Here's how the part is built. I have some questions about the finished solid (model axes, mm). Give positions to 0.01 mm unless a question says otherwise; leave off trailing zeros. Write each loop counter-clockwise with the first axis right and the second up, starting at its lowest first coordinate (ties: lowest second). Pieces come first, ordered by that corner, then holes. Notation, with made-up numbers: (48.25, -10) - (55.25, -10) arc R19 cw to (55.25, 8) - close; hole circle Ø5 at (-4, 16.5). An arc over 180 degrees is marked (long way). One line per item, written item: value. Start each with the question number.
1) I'm going to push flat-ended pins straight in: P1, Ø3, axis at y = 82.5, z = 0.5, coming from the +X side; P2, Ø2.5, axis at y = 65.5, z = 1.5, coming from the +X side; P3, Ø1.5, axis at x = 11, z = 3, coming from the +Y side. Where does each tip first touch, or does it pass through?
2) Imagine slicing it at A-A on z = 2.65. Write out the boundary of the cut face in (x, y).
3) Imagine slicing it at B-B on y = 16.5. Write out the boundary of the cut face in (x, z).
4) Imagine slicing it at C-C on x = -57. Write out the boundary of the cut face in (y, z), plus the area to 3 significant figures.
5) Please list where these lines run through material, in increasing order: L1, parallel to X at y = 4.5, z = 2.5; L2, parallel to X at y = 26.5, z = 2.9; L3, parallel to X at y = 55, z = 1.4. Write a range as [from, to].
6) Imagine slicing it at D-D on x = 2. Write out the boundary of the cut face in (y, z), plus the area to 3 significant figures.
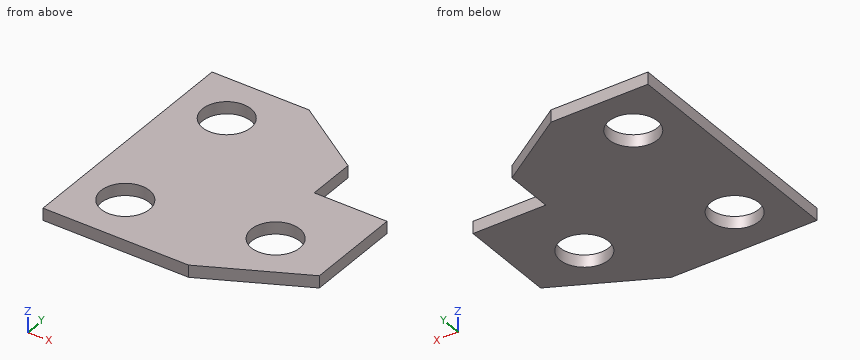
from build123d import *

# Parameters (mm, degrees)
SKETCH1_R           = 10
BOSS_EXTRUDE1_DEPTH = 5


with BuildPart() as part:
    # Sketch1 → Boss-Extrude1 (new body)
    with BuildSketch(Plane.XY):
        Polygon((-73.294117647, 93.764705882), (-73.294117647, -6.235294118), (-13.294117647, -6.235294118), (26.705882353, 13.764705882), (26.705882353, 53.764705882), (-3.294117647, 53.764705882), (-3.294117647, 73.764705882), (-33.294117647, 93.764705882), align=None)
        with Locations((-53.294117647, 73.764705882)):
            Circle(SKETCH1_R, mode=Mode.SUBTRACT)
        with Locations((-53.294117647, 13.764705882)):
            Circle(SKETCH1_R, mode=Mode.SUBTRACT)
        with Locations((1.705882353, 23.764705882)):
            Circle(SKETCH1_R, mode=Mode.SUBTRACT)
    extrude(amount=BOSS_EXTRUDE1_DEPTH)


solid = part.part
Numbers:
1. P1: x = -14.15
1. P2: x = -3.29
1. P3: y = 53.76
2. outline: (-73.29, -6.24) - (-13.29, -6.24) - (26.71, 13.76) - (26.71, 53.76) - (-3.29, 53.76) - (-3.29, 73.76) - (-33.29, 93.76) - (-73.29, 93.76) - close; hole circle Ø20 at (-53.29, 13.76); hole circle Ø20 at (-53.29, 73.76); hole circle Ø20 at (1.71, 23.76)
3. outline: (-73.29, 0) - (-62.91, 0) - (-62.91, 5) - (-73.29, 5) - close; (-43.68, 0) - (-5.17, 0) - (-5.17, 5) - (-43.68, 5) - close; (8.58, 0) - (26.71, 0) - (26.71, 5) - (8.58, 5) - close
4. outline: (-6.24, 0) - (4.48, 0) - (4.48, 5) - (-6.24, 5) - close; (23.05, 0) - (64.48, 0) - (64.48, 5) - (23.05, 5) - close; (83.05, 0) - (93.76, 0) - (93.76, 5) - (83.05, 5) - close
4. area: 314 mm^2
5. L1: [-73.29, -57.06], [-49.53, 8.18]
5. L2: [-73.29, -7.91], [11.32, 26.71]
5. L3: [-73.29, -3.29]
6. outline: (1.41, 0) - (13.77, 0) - (13.77, 5) - (1.41, 5) - close; (33.76, 0) - (53.76, 0) - (53.76, 5) - (33.76, 5) - close
6. area: 162 mm^2
